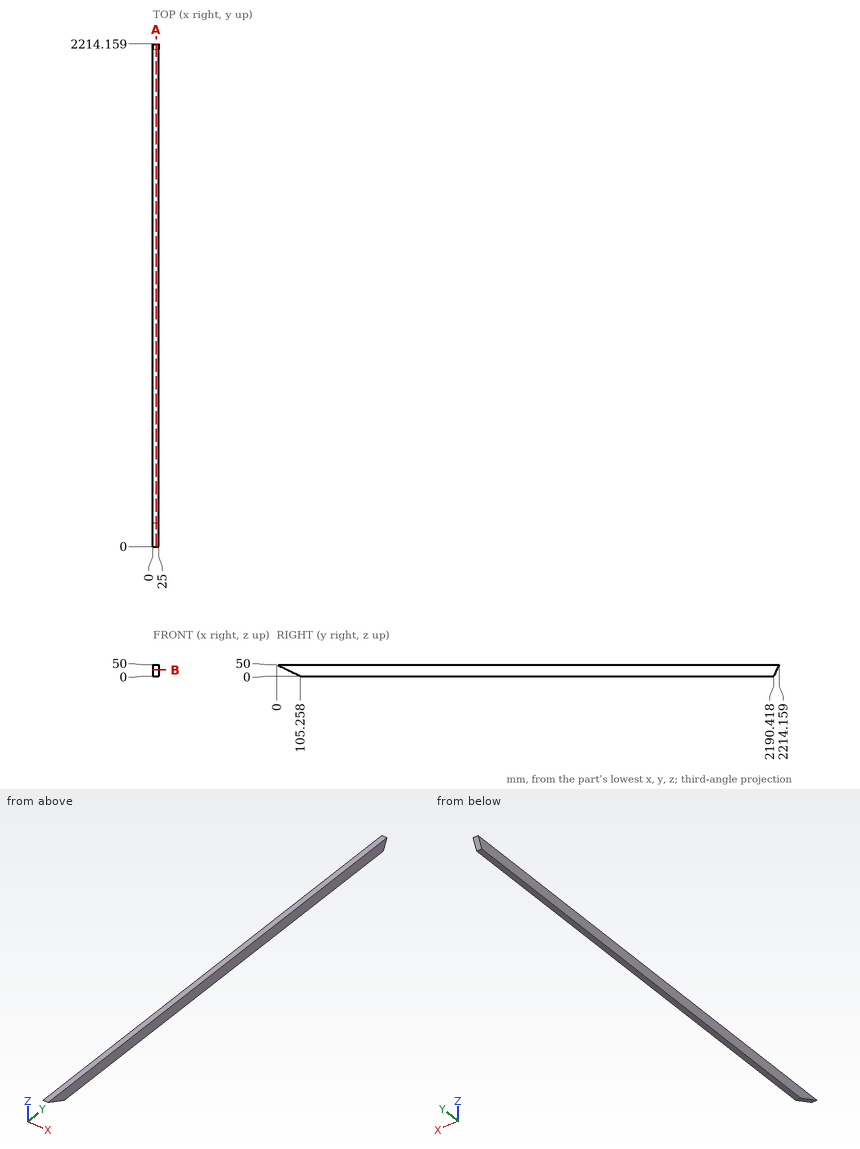
Could you check a few things on this drawing? It's one solid part, dimensions in mm from its lowest x, y, z. Round coordinates to 2 decimals unless told otherwise and drop trailing zeros. Order: outer loops, then holes, each group sorted by start corner. A loop starts at its lowest first (then second) coordinate and runs counter-clockwise, first axis right, second up.
Q1. Please list where these lines run through material, in increasing order: probe 1 along Y at (x, z) = (18.75, 8) (1 decimal); probe 2 along Y at (x, z) = (1.5, 7.5).
Geometry says:
probe 1: y = 88.4 to 2194.2
probe 2: y = 89.47 to 2193.98
Q2. Imagine slicing it at A-A, the plane x = 14. List the corners of the cut face in (y, z) for me.
Geometry says:
outline: (0, 50) - (105.26, 0) - (2190.42, 0) - (2214.16, 50) - close
Q3. I'm going to push flat-ended pins straight in: P1, Ø4, axis at x = 21, z = 16, coming from the -Y side (1 decimal); P2, Ø4, axis at x = 11.5, z = 5.5, coming from the +Y side; P3, Ø3, axis at x = 5.5, z = 36, coming from the -Y side (1 decimal). Where does each tip first touch, or does it pass through?
Geometry says:
P1: stops at y = 67.4
P2: stops at y = 2193.98
P3: stops at y = 26.3
Q4. Imagine slicing it at B-B, the plane z = 27. List the corners of the cut face in (x, y) for me, then the cut area to 3 significant figures.
Geometry says:
outline: (0, 48.42) - (25, 48.42) - (25, 2203.24) - (0, 2203.24) - close
area: 53,900 mm2
